from build123d import *

# Parameters (mm, degrees)
SKETCH1_W             = 50.8
SKETCH1_H             = 101.6
BOSS_EXTRUDE1_DEPTH   = 1.5875
F_8_CLEARANCE_HOLE1_D = 4.3053
SKETCH4_W             = 64.445768018
SKETCH4_H             = 114.740745706
CUT_EXTRUDE1_DEPTH    = 3.175


with BuildPart() as part:
    # Sketch1 → Boss-Extrude1 (new, symmetric)
    with BuildSketch(Plane(origin=(0, 0, 0), x_dir=(0, 0, -1), z_dir=(1, 0, 0))):
        Rectangle(SKETCH1_W, SKETCH1_H)
    extrude(amount=BOSS_EXTRUDE1_DEPTH, both=True)

    # #8 Clearance Hole1 (through all)
    with Locations(Plane.ZY.offset(1.5875)):
        with Locations((-12.7, -41.275), (-12.7, -9.525), (-20.6375, 6.35), (0, 6.35), (12.7, 25.4), (0, 44.45), (-20.6375, 44.45)):
            Hole(F_8_CLEARANCE_HOLE1_D / 2)

    # Sketch4 → Cut-Extrude1 (cut)
    with BuildSketch(Plane.ZY.offset(1.5875)):
        Rectangle(SKETCH4_W, SKETCH4_H)
        with BuildLine():
            Line((-19.05, 50.8), (0, 50.8))
            ThreePointArc((0, 50.8), (2.996297827, 50.048633702), (5.283519369, 47.972346246))
            Line((5.283519369, 47.972346246), (17.983519369, 28.922346246))
            ThreePointArc((17.983519369, 28.922346246), (19.010206024, 26.109788659), (18.633997117, 23.13942967))
            Line((18.633997117, 23.13942967), (-6.766002883, -43.53557033))
            ThreePointArc((-6.766002883, -43.53557033), (-13.434053527, -47.582429383), (-18.994539095, -42.112423182))
            Line((-18.994539095, -42.112423182), (-25.358404321, 5.721932613))
            ThreePointArc((-25.358404321, 5.721932613), (-25.389589702, 6.03527836), (-25.4, 6.35))
            Line((-25.4, 6.35), (-25.4, 44.45))
            ThreePointArc((-25.4, 44.45), (-23.540128061, 48.940128061), (-19.05, 50.8))
        make_face(mode=Mode.SUBTRACT)
    extrude(amount=-CUT_EXTRUDE1_DEPTH, mode=Mode.SUBTRACT)


solid = part.part
Can you work these out from the model? Positions are in its coordinate system, mm. Give positions to 0.01 mm unless a question says otherwise; leave off trailing zeros. Order: outer loops, then holes, each group sorted by start corner. A loop starts at its lowest first (then second) coordinate and runs counter-clockwise, first axis right, second up. Notation, with made-up numbers: M -24,-6.5 L -17,-6.5 A9 ccw -17,8.5 Z; hole C -16,39 d2. An arc over 180 degrees is marked long. Use a Markdown table: item, result. Add a question column.
Item 1: If I drill on L1, parallel to Y at x = -0.8, z = -12.7 (3 decimals); L2, parallel to Z at x = -0.75, y = 42.5; L3, parallel to Y at x = 1.15, z = -14, over which ranges is the centre line in solid material (lowest first)? Write a range as [from, to].
Item 2: Suppose I cut it at B-B (z = 12.7). List the corners of the cut face in (x, y) for me.
Item 3: Suppose I cut it at D-D (x = -0.3). Count the separate pieces of the cut face and the enclosed holes in it, then the cut area to 3 significant figures.
Item 4: Will these pins go through, and if not, where does the flat tip stop? pin 1 (5.5 mm diameter, centred on y = -41.275, z = -12.7, fed in from -X); pin 2 (1 mm diameter, centred on x = 0.5, y = -33, fed in from -Z); pin 3 (1 mm diameter, centred on x = -0.5, z = -21, fed in from +Y); pin 4 (1 mm diameter, centred on x = -1, y = -13, fed in from +Z).
Item 5: Suppose I cut it at C-C (z = -11.5). List the corners of the cut face in (x, y) for me.
Item 6: Suppose I cut it at A-A (y = 25.4). List the corners of the cut face in (x, z) for me.
Item 7: We'd pull the mould along Y, two halves only. Please class faces 1 (the flat face through (-0.022, -9.731, 6.112)), 2 (the cylindrical face through (0.02, 4.25, 0.47)), 3 (the flat face through (-0.022, 38.581, 11.545)): +Y half, -Y half, draft (parallel to the pull), parting line (faces both ways), or undercut.
Answer sheet:
| question | item | result |
|---|---|---|
| 1 | L1 | y = [-47.625, -43.428], [-39.122, -11.678], [-7.372, 50.8] |
| 1 | L2 | z = [-25.4, -21.55], [-19.73, -0.91], [0.91, 8.93] |
| 1 | L3 | y = [-47.49, -42.99], [-39.56, -11.24], [-7.81, 50.8] |
| 2 | outline | M -1.59,7.56 L 1.59,7.56 L 1.59,23.25 L -1.59,23.25 Z; M -1.59,27.55 L 1.59,27.55 L 1.59,36.85 L -1.59,36.85 Z |
| 3 | separate pieces | 1 |
| 3 | enclosed holes | 7 |
| 3 | area | 2,890 mm² |
| 4 | pin 1 | stops at x = -1.59 |
| 4 | pin 2 | stops at z = -20.27 |
| 4 | pin 3 | stops at y = 50.63 |
| 4 | pin 4 | stops at z = 5.06 |
| 5 | outline | M -1.59,-47.51 L 1.59,-47.51 L 1.59,-43.06 L -1.59,-43.06 Z; M -1.59,-39.49 L 1.59,-39.49 L 1.59,-11.31 L -1.59,-11.31 Z; M -1.59,-7.74 L 1.59,-7.74 L 1.59,50.8 L -1.59,50.8 Z |
| 6 | outline | M -1.59,-25.4 L 1.59,-25.4 L 1.59,10.55 L -1.59,10.55 Z; M -1.59,14.85 L 1.59,14.85 L 1.59,19.05 L -1.59,19.05 Z |
| 7 | face 1 | -Y half |
| 7 | face 2 | undercut |
| 7 | face 3 | +Y half |
